CAD build for the part. Positions are in the model's coordinates, mm. A direction names the side the tool comes from. Give positions to 0.01 mm unless a question says otherwise; leave off trailing zeros. Loops run counter-clockwise (first coordinate to the right, second up) from the corner with the lowest first, then second, coordinate; pieces in that order, holes last.
Item 1: Which spindle directions (+Z, -Z, +X, -X, +Y, -Y) get a long thin tool onto all of the face, cutting with end or side? Do faces 1 (the flat face through (-1, -11.598, 2)), 2 (the flat face through (-22.833, 11, 2)), 3 (the cylindrical face through (-19.911, -8.696, 2.522)), 4 (the flat face through (-22.833, -6, 2)), 5 (the flat face through (20.855, 10, 2)). Say none if no direction does.
Item 2: Saw through at D-D on x = 19. Give the cut face in (y, z).
Item 3: Drop flat-ended pins along their axis: P1, Ø1.9, axis at y = 8.5, z = 3, coming from the -X side; P2, Ø2, axis at y = 0, z = 2, coming from the +X side; P3, Ø1, axis at y = -8.5, z = 1.5, coming from the +X side. Give the stop position or say it passes through.
Item 4: Probe probe 1 along Y at (x, z) = (-13, 2.3); probe 2 along X at (y, z) = (2.5, 0.65); probe 3 along X at (y, z) = (12.5, 2.2). List the from-to ranges inside material, lowest first.
Item 5: Saw through at B-B on x = 1. Give the cut face in (y, z).
Item 6: Saw through at C-C on y = 11.75. Give the cut face in (x, z).
Item 7: Saw through at A-A on z = 0.8. Give the cut face in (x, y).
from build123d import *

# Parameters (mm, degrees)
F0_W     = 43.688
F0_H     = 27.94
F1_DEPTH = 3.81
F2_DEPTH = 1.27
F4_DEPTH = 3.81
F3_R     = 2.54
F5_DEPTH = 25.4


with BuildPart() as f1:
    # F0 (on Top) → F1 (new body)
    with BuildSketch(Plane.XY):
        with Locations((-0.9886939079, 2.3718496937)):
            Rectangle(F0_W, F0_H)
        with BuildLine():
            ThreePointArc((-20.2926939079, 12.5318496937), (-19.92071952, 13.4298753058), (-19.0226939079, 13.8018496937))
            Line((-19.0226939079, 13.8018496937), (17.0453060921, 13.8018496937))
            ThreePointArc((17.0453060921, 13.8018496937), (17.9433317042, 13.4298753058), (18.3153060921, 12.5318496937))
            Line((18.3153060921, 12.5318496937), (18.3153060921, 9.9918496937))
            ThreePointArc((18.3153060921, 9.9918496937), (17.9433317042, 9.0938240816), (17.0453060921, 8.7218496937))
            Line((17.0453060921, 8.7218496937), (14.7593060921, 8.7218496937))
            ThreePointArc((14.7593060921, 8.7218496937), (13.86128048, 8.3498753058), (13.4893060921, 7.4518496937))
            Line((13.4893060921, 7.4518496937), (13.4893060921, -2.4541503063))
            ThreePointArc((13.4893060921, -2.4541503063), (13.86128048, -3.3521759184), (14.7593060921, -3.7241503063))
            Line((14.7593060921, -3.7241503063), (17.0453060921, -3.7241503063))
            ThreePointArc((17.0453060921, -3.7241503063), (17.9433317042, -4.0961246942), (18.3153060921, -4.9941503063))
            Line((18.3153060921, -4.9941503063), (18.3153060921, -7.7881503063))
            ThreePointArc((18.3153060921, -7.7881503063), (17.9433317042, -8.6861759184), (17.0453060921, -9.0581503063))
            Line((17.0453060921, -9.0581503063), (-19.0226939079, -9.0581503063))
            ThreePointArc((-19.0226939079, -9.0581503063), (-19.92071952, -8.6861759184), (-20.2926939079, -7.7881503063))
            Line((-20.2926939079, -7.7881503063), (-20.2926939079, -5.2481503063))
            ThreePointArc((-20.2926939079, -5.2481503063), (-19.92071952, -4.3501246942), (-19.0226939079, -3.9781503063))
            Line((-19.0226939079, -3.9781503063), (-16.7366939079, -3.9781503063))
            ThreePointArc((-16.7366939079, -3.9781503063), (-15.8386682958, -3.6061759184), (-15.4666939079, -2.7081503063))
            Line((-15.4666939079, -2.7081503063), (-15.4666939079, 7.1978496937))
            ThreePointArc((-15.4666939079, 7.1978496937), (-15.8386682958, 8.0958753058), (-16.7366939079, 8.4678496937))
            Line((-16.7366939079, 8.4678496937), (-19.0226939079, 8.4678496937))
            ThreePointArc((-19.0226939079, 8.4678496937), (-19.92071952, 8.8398240816), (-20.2926939079, 9.7378496937))
            Line((-20.2926939079, 9.7378496937), (-20.2926939079, 12.5318496937))
        make_face(mode=Mode.SUBTRACT)
    extrude(amount=F1_DEPTH)

    # F0 (on Top) → F2 (join)
    with BuildSketch(Plane.XY):
        with BuildLine():
            Line((17.0453060921, 13.8018496937), (-19.0226939079, 13.8018496937))
            ThreePointArc((-19.0226939079, 13.8018496937), (-19.92071952, 13.4298753058), (-20.2926939079, 12.5318496937))
            Line((-20.2926939079, 12.5318496937), (-20.2926939079, 9.7378496937))
            ThreePointArc((-20.2926939079, 9.7378496937), (-19.92071952, 8.8398240816), (-19.0226939079, 8.4678496937))
            Line((-19.0226939079, 8.4678496937), (-16.7366939079, 8.4678496937))
            ThreePointArc((-16.7366939079, 8.4678496937), (-15.8386682958, 8.0958753058), (-15.4666939079, 7.1978496937))
            Line((-15.4666939079, 7.1978496937), (-15.4666939079, -2.7081503063))
            ThreePointArc((-15.4666939079, -2.7081503063), (-15.8386682958, -3.6061759184), (-16.7366939079, -3.9781503063))
            Line((-16.7366939079, -3.9781503063), (-19.0226939079, -3.9781503063))
            ThreePointArc((-19.0226939079, -3.9781503063), (-19.92071952, -4.3501246942), (-20.2926939079, -5.2481503063))
            Line((-20.2926939079, -5.2481503063), (-20.2926939079, -7.7881503063))
            ThreePointArc((-20.2926939079, -7.7881503063), (-19.92071952, -8.6861759184), (-19.0226939079, -9.0581503063))
            Line((-19.0226939079, -9.0581503063), (17.0453060921, -9.0581503063))
            ThreePointArc((17.0453060921, -9.0581503063), (17.9433317042, -8.6861759184), (18.3153060921, -7.7881503063))
            Line((18.3153060921, -7.7881503063), (18.3153060921, -4.9941503063))
            ThreePointArc((18.3153060921, -4.9941503063), (17.9433317042, -4.0961246942), (17.0453060921, -3.7241503063))
            Line((17.0453060921, -3.7241503063), (14.7593060921, -3.7241503063))
            ThreePointArc((14.7593060921, -3.7241503063), (13.86128048, -3.3521759184), (13.4893060921, -2.4541503063))
            Line((13.4893060921, -2.4541503063), (13.4893060921, 7.4518496937))
            ThreePointArc((13.4893060921, 7.4518496937), (13.86128048, 8.3498753058), (14.7593060921, 8.7218496937))
            Line((14.7593060921, 8.7218496937), (17.0453060921, 8.7218496937))
            ThreePointArc((17.0453060921, 8.7218496937), (17.9433317042, 9.0938240816), (18.3153060921, 9.9918496937))
            Line((18.3153060921, 9.9918496937), (18.3153060921, 12.5318496937))
            ThreePointArc((18.3153060921, 12.5318496937), (17.9433317042, 13.4298753058), (17.0453060921, 13.8018496937))
        make_face()
    extrude(amount=F2_DEPTH)

    # F3 (on face) → F4 (join)
    with BuildSketch(Plane.XY.offset(3.81)):
        with BuildLine():
            Line((-22.8326939079, -0.3490345376), (-22.8326939079, 5.092733925))
            ThreePointArc((-22.8326939079, 5.092733925), (-23.9756939079, 2.3718496937), (-22.8326939079, -0.3490345376))
        make_face()
        with BuildLine():
            ThreePointArc((21.7443060921, 2.3718496937), (21.5151656258, 3.673212441), (20.8553060921, 4.8180424498))
            Line((20.8553060921, 4.8180424498), (20.8553060921, -0.0743430624))
            ThreePointArc((20.8553060921, -0.0743430624), (21.5151656258, 1.0704869464), (21.7443060921, 2.3718496937))
        make_face()
    extrude(amount=-F4_DEPTH)

    # F3 (on face) → F5 (cut)
    with BuildSketch(Plane.XY.offset(3.81)):
        with Locations((-20.1656939079, 2.3718496937)):
            Circle(F3_R)
        with Locations((17.9343060921, 2.3718496937)):
            Circle(F3_R)
    extrude(amount=-F5_DEPTH, mode=Mode.SUBTRACT)


solid = f1.part
Results below:
1. face 1: +Z, -Z, +X, -X, -Y
1. face 2: +Z, -Z, -X, +Y
1. face 3: +Z
1. face 4: +Z, -Z, -X, -Y
1. face 5: +Z, -Z, +X, +Y
2. outline: (-11.6, 0) - (0.07, 0) - (0.07, 3.81) - (-11.6, 3.81) - close; (4.68, 0) - (16.34, 0) - (16.34, 3.81) - (4.68, 3.81) - close
3. P1: stops at x = -22.83
3. P2: stops at x = 21.49
3. P3: stops at x = 20.86
4. probe 1: y = -11.6 to -9.06, 13.8 to 16.34
4. probe 2: x = -23.97 to -22.7, -17.63 to 15.4, 20.47 to 21.74
4. probe 3: x = -22.83 to -20.29, 18.32 to 20.86
5. outline: (-11.6, 0) - (16.34, 0) - (16.34, 3.81) - (13.8, 3.81) - (13.8, 1.27) - (-9.06, 1.27) - (-9.06, 3.81) - (-11.6, 3.81) - close
6. outline: (-22.83, 0) - (20.86, 0) - (20.86, 3.81) - (18.32, 3.81) - (18.32, 1.27) - (-20.29, 1.27) - (-20.29, 3.81) - (-22.83, 3.81) - close
7. outline: (-22.83, -11.6) - (20.86, -11.6) - (20.86, -0.07) arc R3.81 ccw to (20.86, 4.82) - (20.86, 16.34) - (-22.83, 16.34) - (-22.83, 5.09) arc R3.81 ccw to (-22.83, -0.35) - close; hole circle Ø5.08 at (-20.17, 2.37); hole circle Ø5.08 at (17.93, 2.37)
